Autodesk Inventor part; units mm, degrees
ref_plane "YZ Plane" through (0, 0, 0) normal (1, 0, 0) x (0, 1, 0)
ref_plane "XZ Plane" through (0, 0, 0) normal (0, 1, 0) x (-1, 0, 0)
ref_plane "XY Plane" through (0, 0, 0) normal (0, 0, 1) x (1, 0, 0)
sketch "Sketch1" plane through (0, 0, 0) normal (0, 0, 1) x (1, 0, 0)
  line L0 (30.1319, -27.3816) -> (15.1319, -27.3816)
  line L1 (15.1319, -27.3816) -> (15.1319, -32.3816)
  line L2 (15.1319, -32.3816) -> (30.1319, -32.3816)
  line L3 (30.1319, -32.3816) -> (30.1319, -27.3816)
  point P0 (0, 0)
  dimension "d0" = 15
  dimension "d1" = 5
extrude "Extrusion1" add sketch "Sketch1" along normal blind 10
fillet "Fillet1" radius 4 2 edges at (15.1319, -29.8816, 10) (30.1319, -29.8816, 10)
sketch "Sketch2" plane through (15.1319, -27.3816, 0) normal (0, 1, 0) x (1, 0, 0)
  circle A0 centre (7.5, -5) radius 2
  line L0 (11, -10) -> (4, -10)
  line L1 (0, 0) -> (0, -6)
  point P0 (-15.1319, 0)
  dimension "d5" = 4
  dimension "d6" = 5
  dimension "d7" = 7.5
extrude "Extrusion2" cut sketch "Sketch2" against normal blind 7.5
thread "Thread1"
properties part number "víko_držák" material "Aluminum 6061"
The listing builds one solid part. Answer for the finished solid, in the listing's coordinates (mm). Give positions to 0.01 mm unless a question says otherwise; leave off trailing zeros. Write each loop counter-clockwise with the first axis right and the second up, starting at its lowest first coordinate (ties: lowest second). Pieces come first, ordered by that corner, then holes. Notation, with made-up numbers: (21, 51.5) - (59, 51.5) arc R28 cw to (59, 87.5) - close; hole circle Ø10 at (-22.5, 15). An arc over 180 degrees is marked (long way). Use a Markdown table: item, result.
1. Section C-C on z = 3.5 is taken. Write down the section's boundary in (x, y), plus the area to 3 significant figures.
Values follow:
| item | result |
|---|---|
| outline | (15.13, -32.38) - (21.31, -32.38) - (21.31, -27.38) - (15.13, -27.38) - close; (23.95, -32.38) - (30.13, -32.38) - (30.13, -27.38) - (23.95, -27.38) - close |
| area | 61.8 mm² |
2. Section B-B on y = -27.8 is taken. Write down the section's boundary in (x, z), plus the area to 3 significant figures.
Values follow:
| item | result |
|---|---|
| outline | (15.13, 0) - (30.13, 0) - (30.13, 6) arc R4 ccw to (26.13, 10) - (19.13, 10) arc R4 ccw to (15.13, 6) - close; hole circle Ø4 at (22.63, 5) |
| area | 131 mm² |
3. Section A-A on z = 5 is taken. Write down the section's boundary in (x, y), plus the area to 3 significant figures.
Values follow:
| item | result |
|---|---|
| outline | (15.13, -32.38) - (20.63, -32.38) - (20.63, -27.38) - (15.13, -27.38) - close; (24.63, -32.38) - (30.13, -32.38) - (30.13, -27.38) - (24.63, -27.38) - close |
| area | 55.0 mm² |
4. Find the intervals of material crossed by probe 1 along Z at (x, y) = (22.75, -30.8); probe 2 along X at (y, z) = (-29.6, 5); probe 3 along X at (y, z) = (-28.3, 3.25), in increasing order. Write a range as from..to.
Values follow:
| item | result |
|---|---|
| probe 1 | z = 0..3, 7..10 |
| probe 2 | x = 15.13..20.63, 24.63..30.13 |
| probe 3 | x = 15.13..21.66, 23.6..30.13 |
5. Section D-D on x = 28.75 is taken. Write down the section's boundary in (y, z).
Values follow:
| item | result |
|---|---|
| outline | (-32.38, 0) - (-27.38, 0) - (-27.38, 9.02) - (-32.38, 9.02) - close |
